```python
from build123d import *

# Parameters (mm, degrees)
SKETCH1_W           = 25.4
SKETCH1_H           = 50.8
SKETCH1_W_2         = 18.9992
SKETCH1_H_2         = 44.3992
BOSS_EXTRUDE1_DEPTH = 749.3
SKETCH2_W           = 25.4
SKETCH2_H           = 50.8
CUT_EXTRUDE1_DEPTH  = 393.7
SKETCH3_W           = 25.4
SKETCH3_H           = 50.8
CUT_EXTRUDE2_DEPTH  = 393.7


with BuildPart() as part:
    # Sketch1 → Boss-Extrude1 (new, symmetric)
    with BuildSketch(Plane.XY):
        Rectangle(SKETCH1_W, SKETCH1_H)
        Rectangle(SKETCH1_W_2, SKETCH1_H_2, mode=Mode.SUBTRACT)
    extrude(amount=BOSS_EXTRUDE1_DEPTH, both=True)

    # Sketch2 → Cut-Extrude1 (cut)
    with BuildSketch(Plane.XY.offset(749.3)):
        Rectangle(SKETCH2_W, SKETCH2_H)
    extrude(amount=-CUT_EXTRUDE1_DEPTH, mode=Mode.SUBTRACT)

    # Sketch3 → Cut-Extrude2 (cut)
    with BuildSketch(Plane(origin=(0, 0, -749.3), x_dir=(-1, 0, 0), z_dir=(0, 0, -1))):
        Rectangle(SKETCH3_W, SKETCH3_H)
    extrude(amount=-CUT_EXTRUDE2_DEPTH, mode=Mode.SUBTRACT)


solid = part.part
```
Part model, mm, in its own coordinate system. A direction names the side the tool comes from. Coordinates: 2 decimals unless noted, no trailing zeros. Order: outer loops, then holes, each group sorted by start corner. A loop starts at its lowest first (then second) coordinate and runs counter-clockwise, first axis right, second up. Notation, with made-up numbers: (-13.75, 50) -> (40.25, 50) arc R18 cw to (40.25, 61) -> close; hole circle Ø7 at (5, 79.25). An arc over 180 degrees is marked (long way). Put each result on its own line as item: value. Start each with the question number.
(1) Band-saw the part on A-A (z = -108). Give the cut face in (x, y).
(2) Probe line 1 along Y through (x, z) = (5.5, 112.5); line 2 along X through (y, z) = (3, -48.5). List the from-to ranges inside material, lowest first. Write a range as [from, to].
(3) Mould opens along Y. For faces 1 (the face through (0, 25.4, 5)), 2 (the face through (-11, 0, -355.6)), 3 (the face through (-9.5, 0, 5)) say: pulls with the +Y half, pulls with the -Y half, needs draft (parallel to the pull), parting line crosses it, or undercut.
(4) Band-saw the part on B-B (x = -2.75). Give the cut face in (y, z), then the cut area to 3 significant figures.
(5) Which spindle directions (+Z, -Z, +X, -X, +Y, -Y) get a long thin tool onto all of the face, cutting with end or side? Do faces 4 (the face through (0, -22.2, 5)), 5 (the face through (12.7, 0, 5)). Say none if no direction does.
(6) Band-saw the part on C-C (y = 7). Give the cut face in (x, z), then the cut area to 3 significant figures.
Determined:
1. outline: (-12.7, -25.4) -> (12.7, -25.4) -> (12.7, 25.4) -> (-12.7, 25.4) -> close; hole (-9.5, -22.2) -> (9.5, -22.2) -> (9.5, 22.2) -> (-9.5, 22.2) -> close
2. line 1: y = [-25.4, -22.2], [22.2, 25.4]
2. line 2: x = [-12.7, -9.5], [9.5, 12.7]
3. face 1: pulls with the +Y half
3. face 2: needs draft
3. face 3: undercut
4. outline: (-25.4, -355.6) -> (-22.2, -355.6) -> (-22.2, 355.6) -> (-25.4, 355.6) -> close; (22.2, -355.6) -> (25.4, -355.6) -> (25.4, 355.6) -> (22.2, 355.6) -> close
4. area: 4,550 mm²
5. face 4: +Z, -Z
5. face 5: +Z, -Z, +X, +Y, -Y
6. outline: (-12.7, -355.6) -> (-9.5, -355.6) -> (-9.5, 355.6) -> (-12.7, 355.6) -> close; (9.5, -355.6) -> (12.7, -355.6) -> (12.7, 355.6) -> (9.5, 355.6) -> close
6. area: 4,550 mm²
